Autodesk Inventor part; units mm, degrees
ref_plane "Work Plane2" through (-70.375, 15.375, 4.7) normal (0, 0, -1) x (0, 1, 0)
ref_plane "Work Plane3" through (-14.375, -14.375, -5) normal (0, 0, 1) x (1, 0, 0)
ref_plane "YZ Plane" through (0, 0, 0) normal (1, 0, 0) x (0, 1, 0)
ref_plane "Work Plane1" through (0, 0, 0) normal (0, 0, 1) x (1, 0, 0)
sketch "Sketch1" plane through (0, 0, 0) normal (0, 0, 1) x (1, 0, 0)
  circle A0 centre (8, 0) radius 1.0564
  circle A1 centre (-8, 0) radius 1.0564
  circle A2 centre (0, 0) radius 5
  circle A3 centre (0, 0) radius 13.7
  line L0 (-18.375, 15.375) -> (-18.375, 1)
  line L1 (-18.375, 1) -> (-13.6635, 1)
  arc A4 (13.6635, 1) -> (-13.6635, 1) centre (0, 0) ccw
  line L2 (13.6635, 1) -> (18.1635, 1)
  line L3 (18.1635, 1) -> (18.1635, 15.375)
  line L4 (18.1635, 15.375) -> (-18.375, 15.375)
  line L5 (18.1635, 15.375) -> (-18.375, 15.375)
  line L6 (-18.375, 15.375) -> (-18.375, -3.0565)
  line L7 (-18.375, -3.0565) -> (18.1635, -3.0565)
  line L8 (18.1635, -3.0565) -> (18.1635, 15.375)
  line L9 (18.1635, -5.0565) -> (12.7327, -5.0565)
  circle A5 centre (0, 0) radius 6.4423
  arc A6 (2.7565, 5.1523) -> (1.2674, 3.6504) centre (5.3281, 1.1135) ccw
  arc A7 (1.2674, 3.6504) -> (0.6807, 3.8037) centre (0, 0) ccw
  arc A8 (0.6807, 3.8037) -> (0.1169, 5.8421) centre (-4.102, 3.578) ccw
  arc A9 (0.1169, 5.8421) -> (-0.7984, 5.7885) centre (0, 0) ccw
  arc A10 (-0.7984, 5.7885) -> (-1.1203, 3.6981) centre (3.6561, 4.0326) ccw
  arc A11 (-1.1203, 3.6981) -> (-1.685, 3.4774) centre (0, 0) ccw
  arc A12 (-1.685, 3.4774) -> (-3.3393, 4.7951) centre (-5.4217, 0.4836) ccw
  arc A13 (-3.3393, 4.7951) -> (-4.0483, 4.2137) centre (0, 0) ccw
  arc A14 (-4.0483, 4.2137) -> (-3.0801, 2.3334) centre (0.5875, 5.4114) ccw
  arc A15 (-3.0801, 2.3334) -> (-3.4072, 1.8228) centre (0, 0) ccw
  arc A16 (-3.4072, 1.8228) -> (-5.52, 1.9165) centre (-4.6705, -2.7956) ccw
  arc A17 (-5.52, 1.9165) -> (-5.7519, 1.0294) centre (0, 0) ccw
  arc A18 (-5.7519, 1.0294) -> (-3.8633, 0.0773) centre (-2.7054, 4.7233) ccw
  arc A19 (-3.8633, 0.0773) -> (-3.8279, -0.528) centre (0, 0) ccw
  arc A20 (-3.8279, -0.528) -> (-5.5923, -1.6941) centre (-2.1353, -5.0069) ccw
  arc A21 (-5.5923, -1.6941) -> (-5.2584, -2.5481) centre (0, 0) ccw
  arc A22 (-5.2584, -2.5481) -> (-3.171, -2.2083) centre (-4.965, 2.231) ccw
  arc A23 (-3.171, -2.2083) -> (-2.7865, -2.6771) centre (0, 0) ccw
  arc A24 (-2.7865, -2.6771) -> (-3.5285, -4.6576) centre (1.2155, -5.3058) ccw
  arc A25 (-3.5285, -4.6576) -> (-2.7565, -5.1523) centre (0, 0) ccw
  arc A26 (-2.7565, -5.1523) -> (-1.2674, -3.6504) centre (-5.3281, -1.1135) ccw
  arc A27 (-1.2674, -3.6504) -> (-0.6807, -3.8037) centre (0, 0) ccw
  arc A28 (-0.6807, -3.8037) -> (-0.1169, -5.8421) centre (4.102, -3.578) ccw
  arc A29 (-0.1169, -5.8421) -> (0.7984, -5.7885) centre (0, 0) ccw
  arc A30 (0.7984, -5.7885) -> (1.1203, -3.6981) centre (-3.6561, -4.0326) ccw
  arc A31 (1.1203, -3.6981) -> (1.685, -3.4774) centre (0, 0) ccw
  arc A32 (1.685, -3.4774) -> (3.3393, -4.7951) centre (5.4217, -0.4836) ccw
  arc A33 (3.3393, -4.7951) -> (4.0483, -4.2137) centre (0, 0) ccw
  arc A34 (4.0483, -4.2137) -> (3.0801, -2.3334) centre (-0.5875, -5.4114) ccw
  arc A35 (3.0801, -2.3334) -> (3.4072, -1.8228) centre (0, 0) ccw
  arc A36 (3.4072, -1.8228) -> (5.52, -1.9165) centre (4.6705, 2.7956) ccw
  arc A37 (5.52, -1.9165) -> (5.7519, -1.0294) centre (0, 0) ccw
  arc A38 (5.7519, -1.0294) -> (3.8633, -0.0773) centre (2.7054, -4.7233) ccw
  arc A39 (3.8633, -0.0773) -> (3.8279, 0.528) centre (0, 0) ccw
  arc A40 (3.8279, 0.528) -> (5.5923, 1.6941) centre (2.1353, 5.0069) ccw
  arc A41 (5.5923, 1.6941) -> (5.2584, 2.5481) centre (0, 0) ccw
  arc A42 (5.2584, 2.5481) -> (3.171, 2.2083) centre (4.965, -2.231) ccw
  arc A43 (3.171, 2.2083) -> (2.7865, 2.6771) centre (0, 0) ccw
  arc A44 (2.7865, 2.6771) -> (3.5285, 4.6576) centre (-1.2155, 5.3058) ccw
  arc A45 (3.5285, 4.6576) -> (2.7565, 5.1523) centre (0, 0) ccw
  point P0 (-5.6711, -3.0565)
  point P1 (-6.9927, -0.3186)
  point P2 (-6.9927, 0.3186)
  point P3 (6.9927, 0.3186)
  point P4 (6.9927, -0.3186)
  point P5 (5.6711, -3.0565)
  point P6 (0.3418, -6.4333)
  point P7 (0.3418, -5.8333)
  dimension "d0" = 2
  dimension "d4" = 0.6
ref_plane "Work Plane2" through (-70.375, 15.375, 4.7) normal (0, 0, -1) x (0, 1, 0)
extrude "Extrusion1" add sketch "Sketch1" along normal up to surface (4.7 mm away) contours A5 L7 A3 | A3 L2 L8 L7 | L7 L6 L1 A3 | A3 L1 L0 L4 L3 L2 picked at (8.5523, 7.2456)
sketch "Sketch2" plane through (0, 0, 0) normal (0, 0, -1) x (-1, 0, 0)
  circle A0 centre (-8, 0) radius 1.0564
  circle A1 centre (8, 0) radius 1.0564
  circle A2 centre (0, 0) radius 5
  circle A3 centre (0, 0) radius 13.7
  line L0 (-5.6711, -3.0565) -> (-18.1635, -3.0565)
  arc A4 (5.6711, -3.0565) -> (-5.6711, -3.0565) centre (0, 0) ccw
  line L1 (18.375, -3.0565) -> (5.6711, -3.0565)
  line L2 (18.375, 15.375) -> (18.375, -3.0565)
  line L3 (-18.1635, 15.375) -> (18.375, 15.375)
  line L4 (-18.1635, -3.0565) -> (-18.1635, 15.375)
  circle A5 centre (-8, 0) radius 1.0564
  circle A6 centre (8, 0) radius 1.0564
  point P0 (-13.3547, -3.0565)
  point P1 (13.3547, -3.0565)
ref_plane "Work Plane3" through (-14.375, -14.375, -5) normal (0, 0, 1) x (1, 0, 0)
extrude "Extrusion2" add sketch "Sketch2" along normal up to surface (5 mm away) contours A3 L0 L4 L3 L2 L1
sketch "Sketch3" plane through (5.6711, -3.0565, 4.7) normal (0, -1, 0) x (1, 0, 0)
  circle A0 centre (10.2923, -6.7) radius 1.8
  circle A1 centre (-21.8461, -6.7) radius 1.8
  point P0 (-5.6711, -4.7)
hole "Hole1" at (15.9635, -3.0565, -2) at (-16.175, -3.0565, -2) direction (0, 1, 0) diameter 3.6 end through all counterbore diameter 11 counterbore depth 0
properties part number "right_motor_floor"
Can you work these out from the model? Positions are in its coordinate system, mm. A direction names the side the tool comes from. Round coordinates to 2 decimals unless told otherwise and drop trailing zeros. Loops run counter-clockwise (first coordinate to the right, second up) from the corner with the lowest first, then second, coordinate; pieces in that order, holes last. Notation, with made-up numbers: (-2, 48.25) - (17, 48.25) arc R13 ccw to (17, 60.25) - close; hole circle Ø11 at (85, 58.5). An arc over 180 degrees is marked (long way). Write item = value, one per line. Start each with the question number.
(1) For P1, Ø10.5, axis at x = 0, y = 0, coming from the +Z side (3 decimals); P2, Ø1, axis at x = 5, y = 6.5, coming from the -Z side, each with a flat end and sliding along its axis, tell me the tip position at first contact or that it passes through.
(2) If we section it at A-A (y = 2.5): Please give me the cut outline in (x, z) (1 decimal), and give its area (3 significant figures).
(3) If we section it at D-D (y = 0): Please give me the cut outline in (x, z) (1 decimal).
(4) If we mould it in two halves opening along X, with no side actions, what happens to faces 3 (the face through (-14.418, 6.288, -1.61)), 4 (the face through (18.164, 6, 0)), 5 (the face through (0, 14, -5))? For each: released by +X, released by -X, zero draft, split by the parting line, or undercut.
(5) For faces 1 (the face through (0.344, 13.696, -2.465)), 2 (the face through (-18.375, 6, 0)), which set-ups out of +Z, -Z, +X, -X, +Y, -Y let a thin tool reach every point of the face, with its end or its side?
(6) If we section it at B-B (x = -8): Please give me the cut outline in (y, z) (1 decimal).
(7) If I drill on probe 1 along X at (y, z) = (10.5, -2) (1 decimal); probe 2 along X at (y, z) = (0, -1.2) (1 decimal); probe 3 along Z at (x, y) = (9.5, -1.25), over which ranges is the centre line in solid material (lowest first)? Write a range as [from, to].
(8) If we section it at C-C (z = -1.5): Please give me the cut outline in (x, y) (1 decimal).
Ans:
q1.P1 = through
q1.P2 = 0
q2.outline = (-18.4, -5) - (-13.5, -5) - (-13.5, 0) - (-5.9, 0) - (-5.9, 4.7) - (-18.4, 4.7) - close; (5.9, 0) - (13.5, 0) - (13.5, -5) - (18.2, -5) - (18.2, 4.7) - (5.9, 4.7) - close; hole circle Ø3.6 at (-16.2, -2); hole circle Ø3.6 at (16, -2)
q2.area = 144 mm²
q3.outline = (-18.4, -5) - (-13.7, -5) - (-13.7, 0) - (-9.1, 0) - (-9.1, 4.7) - (-18.4, 4.7) - close; (-6.9, 0) - (-6.4, 0) - (-6.4, 4.7) - (-6.9, 4.7) - close; (6.4, 0) - (6.9, 0) - (6.9, 4.7) - (6.4, 4.7) - close; (9.1, 0) - (13.7, 0) - (13.7, -5) - (18.2, -5) - (18.2, 4.7) - (9.1, 4.7) - close; hole circle Ø3.6 at (-16.2, -2); hole circle Ø3.6 at (16, -2)
q4.face_3 = undercut
q4.face_4 = released by +X
q4.face_5 = zero draft
q5.face_1 = -Z
q5.face_2 = +Z, -Z, -X, +Y, -Y
q6.outline = (-3.1, 0) - (-1.1, 0) - (-1.1, 4.7) - (-3.1, 4.7) - close; (1.1, 0) - (11.1, 0) - (11.1, -5) - (15.4, -5) - (15.4, 4.7) - (1.1, 4.7) - close
q7.probe_1 = [-18.4, -18], [-14.4, -8.8], [8.8, 14.2], [17.8, 18.2]
q7.probe_2 = [-18.4, -17.8], [-14.6, -13.7], [13.7, 14.4], [17.6, 18.2]
q7.probe_3 = [0, 4.7]
q8.outline = (-18.4, -3.1) - (-17.9, -3.1) - (-17.9, 15.4) - (-18.4, 15.4) - close; (-14.4, -3.1) - (-13.4, -3.1) arc R13.7 cw (long way) to (13.4, -3.1) - (14.2, -3.1) - (14.2, 15.4) - (-14.4, 15.4) - close; (17.7, -3.1) - (18.2, -3.1) - (18.2, 15.4) - (17.7, 15.4) - close
